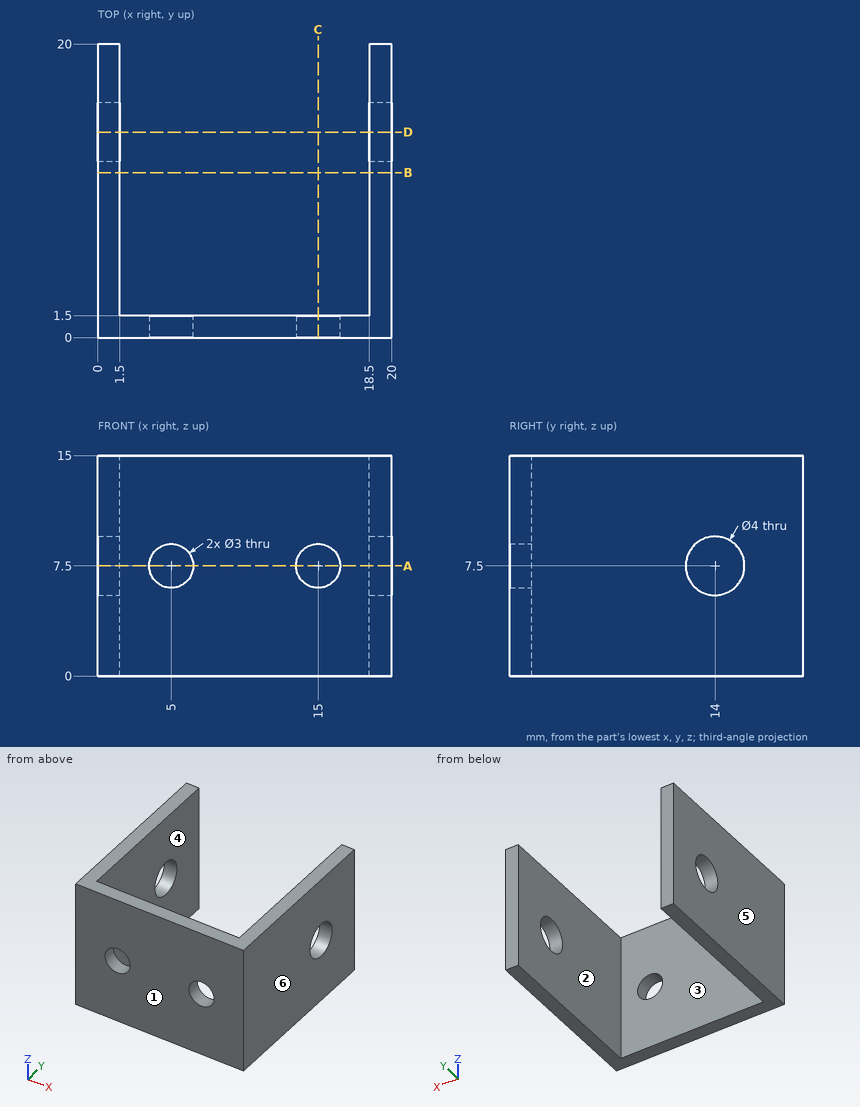
Verification items for this drawing (mm, ordinates from the low corner). A direction names the side the tool comes from. Round coordinates to 2 decimals unless told otherwise and drop trailing zeros. Loops run counter-clockwise (first coordinate to the right, second up) from the corner with the lowest first, then second, coordinate; pieces in that order, holes last. Notation, with made-up numbers: (-39, -29) -> (18, -29) arc R25 ccw to (18, -9) -> close; hole circle Ø1 at (56, -18.75). An arc over 180 degrees is marked (long way). Answer in a Markdown table with one row per item.
Q1. Sectioned sample at A-A on z = 7.5. Enter the section's corners in (x, y), then the cut area to 3 significant figures.
Data:
| item | result |
|---|---|
| outline | (0, 0) -> (3.5, 0) -> (3.5, 1.5) -> (1.5, 1.5) -> (1.5, 12) -> (0, 12) -> close; (0, 16) -> (1.5, 16) -> (1.5, 20) -> (0, 20) -> close; (6.5, 0) -> (13.5, 0) -> (13.5, 1.5) -> (6.5, 1.5) -> close; (16.5, 0) -> (20, 0) -> (20, 12) -> (18.5, 12) -> (18.5, 1.5) -> (16.5, 1.5) -> close; (18.5, 16) -> (20, 16) -> (20, 20) -> (18.5, 20) -> close |
| area | 64.5 mm^2 |
Q2. Sectioned sample at D-D on y = 14. Enter the section's corners in (x, z).
Data:
| item | result |
|---|---|
| outline | (0, 0) -> (1.5, 0) -> (1.5, 5.5) -> (0, 5.5) -> close; (0, 9.5) -> (1.5, 9.5) -> (1.5, 15) -> (0, 15) -> close; (18.5, 0) -> (20, 0) -> (20, 5.5) -> (18.5, 5.5) -> close; (18.5, 9.5) -> (20, 9.5) -> (20, 15) -> (18.5, 15) -> close |
Q3. Thickness scan on L1, parallel to X at y = 3.75, z = 10.25; L2, parallel to Y at x = 3.75, z = 8.5; L3, parallel to Z at x = 18.75, y = 13.75. Record the ranges inside material, lowest first.
Data:
| item | result |
|---|---|
| L1 | x = 0 to 1.5, 18.5 to 20 |
| L2 | y = 0 to 1.5 |
| L3 | z = 0 to 5.52, 9.48 to 15 |
Q4. Sectioned sample at C-C on x = 15. Enter the section's corners in (y, z).
Data:
| item | result |
|---|---|
| outline | (0, 0) -> (1.5, 0) -> (1.5, 6) -> (0, 6) -> close; (0, 9) -> (1.5, 9) -> (1.5, 15) -> (0, 15) -> close |
Q5. Sectioned sample at B-B on y = 11.25. Enter the section's corners in (x, z), then the cut area to 3 significant figures.
Data:
| item | result |
|---|---|
| outline | (0, 0) -> (1.5, 0) -> (1.5, 15) -> (0, 15) -> close; (18.5, 0) -> (20, 0) -> (20, 15) -> (18.5, 15) -> close |
| area | 45.0 mm^2 |
Q6. Release check for a two-part mould opening along X. For the marked faces 3, 4, 5 and 6 record: released by +X, released by -X, zero draft, split by the parting line, or undercut.
Data:
| item | result |
|---|---|
| face 3 | undercut |
| face 4 | undercut |
| face 5 | released by -X |
| face 6 | released by +X |
Q7. Set-up check for the marked faces 1 and 2: record each of +Z, -Z, +X, -X, +Y, -Y from which the full face is reachable in a straight line by a thin tool's end or side.
Data:
| item | result |
|---|---|
| face 1 | +Z, -Z, +X, -X, -Y |
| face 2 | +Z, -Z, +Y |
